from build123d import *

# Parameters (mm, degrees)
EXTRUDE_1_DEPTH     = 3
FILLET_1_R          = 1
EXTRUDE_2_DEPTH     = 12
EXTRUDE_2_TAPER     = 3
FILLET_3_R          = 3
FILLET_4_R          = 3
CUT_EXTRUDE_1_DEPTH = 2.54
SKETCH_5_W          = 0.63
SKETCH_5_H          = 0.63
EXTRUDE_3_DEPTH     = 2.54
CHAMFER_2_SIZE      = 0.2
CHAMFER_3_SIZE      = 0.2
CUT_EXTRUDE_2_DEPTH = 5.08
EXTRUDE_4_DEPTH     = 2.54
SKETCH_8_R          = 1.5
CUT_EXTRUDE_3_DEPTH = 0.1


with BuildPart() as part:
    # 草图1 → 凸台-拉伸1 (new body)
    with BuildSketch(Plane(origin=(0, 0, 0), x_dir=(1, 0, 0), z_dir=(0, 1, 0))):
        with BuildLine():
            ThreePointArc((11.109578501, 22.761132302), (9.268225449, 24.866230509), (6.58350481, 25.65))
            Line((6.58350481, 25.65), (-6.58350481, 25.65))
            ThreePointArc((-6.58350481, 25.65), (-9.268225449, 24.866230509), (-11.109578501, 22.761132302))
            Line((-11.109578501, 22.761132302), (-12.92017347, 18.860908481))
            ThreePointArc((-12.92017347, 18.860908481), (-13.440232827, 18.25183334), (-14.200505299, 18))
            ThreePointArc((-14.200505299, 18), (-16.897924527, 16.767729012), (-18, 14.014550498))
            Line((-18, 14.014550498), (-18, 13.985449502))
            Line((-18, 13.985449502), (-18, -13.985449502))
            Line((-18, -13.985449502), (-18, -14.014550498))
            ThreePointArc((-18, -14.014550498), (-16.897924527, -16.767729012), (-14.200505299, -18))
            ThreePointArc((-14.200505299, -18), (-13.440232827, -18.25183334), (-12.92017347, -18.860908481))
            Line((-12.92017347, -18.860908481), (-11.109578501, -22.761132302))
            ThreePointArc((-11.109578501, -22.761132302), (-9.268225449, -24.866230509), (-6.58350481, -25.65))
            Line((-6.58350481, -25.65), (6.58350481, -25.65))
            ThreePointArc((6.58350481, -25.65), (9.268225449, -24.866230509), (11.109578501, -22.761132302))
            Line((11.109578501, -22.761132302), (12.92017347, -18.860908481))
            ThreePointArc((12.92017347, -18.860908481), (13.440232827, -18.25183334), (14.200505299, -18))
            ThreePointArc((14.200505299, -18), (16.897924527, -16.767729012), (18, -14.014550498))
            Line((18, -14.014550498), (18, 14.014550498))
            ThreePointArc((18, 14.014550498), (16.897924527, 16.767729012), (14.200505299, 18))
            ThreePointArc((14.200505299, 18), (13.440232827, 18.25183334), (12.92017347, 18.860908481))
            Line((12.92017347, 18.860908481), (11.109578501, 22.761132302))
        make_face()
        with BuildLine():
            Line((6, -23.15), (-6, -23.15))
            ThreePointArc((-6, -23.15), (-7.5, -21.65), (-6, -20.15))
            Line((-6, -20.15), (6, -20.15))
            ThreePointArc((6, -20.15), (7.5, -21.65), (6, -23.15))
        make_face(mode=Mode.SUBTRACT)
        with BuildLine():
            ThreePointArc((-6, 20.15), (-7.5, 21.65), (-6, 23.15))
            Line((-6, 23.15), (6, 23.15))
            ThreePointArc((6, 23.15), (7.5, 21.65), (6, 20.15))
            Line((6, 20.15), (-6, 20.15))
        make_face(mode=Mode.SUBTRACT)
    extrude(amount=EXTRUDE_1_DEPTH)

    # 圆角1
    fillet_1_edges = [part.edges().sort_by_distance(p)[0] for p in [
        (-12.014875986, 3, 20.811020391),
        (-9.268225449, 3, 24.866230509),
        (0, 3, 25.65),
        (9.268225449, 3, 24.866230509),
        (12.014875986, 3, 20.811020391),
        (13.440232827, 3, 18.25183334),
        (16.897924527, 3, 16.767729012),
        (18, 3, 0),
        (16.897924527, 3, -16.767729012),
        (13.440232827, 3, -18.25183334),
        (12.014875986, 3, -20.811020391),
        (9.268225449, 3, -24.866230509),
        (0, 3, -25.65),
        (-9.268225449, 3, -24.866230509),
        (-12.014875986, 3, -20.811020391),
        (-13.440232827, 3, -18.25183334),
        (-16.897924527, 3, -16.767729012),
        (-18, 3, 0),
        (-16.897924527, 3, 16.767729012),
        (-13.440232827, 3, 18.25183334),
    ]]
    fillet(fillet_1_edges, radius=FILLET_1_R)

    # 草图2 → 凸台-拉伸2 (add)
    with BuildSketch(Plane(origin=(0, 3, 0), x_dir=(1, 0, 0), z_dir=(0, 1, 0))):
        with BuildLine():
            ThreePointArc((-14.15275961, 17.001140476), (-16.174133919, 16.077709334), (-17, 14.014550498))
            Line((-17, 14.014550498), (-17, -14.014550498))
            ThreePointArc((-17, -14.014550498), (-16.174133919, -16.077709334), (-14.15275961, -17.001140476))
            Line((-14.15275961, -17.001140476), (14.15275961, -17.001140476))
            ThreePointArc((14.15275961, -17.001140476), (16.174133919, -16.077709334), (17, -14.014550498))
            Line((17, -14.014550498), (17, 14.014550498))
            ThreePointArc((17, 14.014550498), (16.174133919, 16.077709334), (14.15275961, 17.001140476))
            Line((14.15275961, 17.001140476), (-14.15275961, 17.001140476))
        make_face()
    extrude(amount=EXTRUDE_2_DEPTH, taper=EXTRUDE_2_TAPER)

    # 圆角3
    # the kernel refuses this fillet: 3 mm, written as the material it takes off along each edge
    with BuildSketch(Plane(origin=(-21.254085444, 15, 16.372247124), x_dir=(0, 0, -1), z_dir=(1, 0, 0))) as fillet_3_piece_1:
        with BuildLine():
            CenterArc((FILLET_3_R * 0.948964566715, -FILLET_3_R), FILLET_3_R, 90, 87)
            Line((-FILLET_3_R * 0.0496649680397, -FILLET_3_R * 0.947664043757), (0, 0))
            Line((0, 0), (FILLET_3_R * 0.948964566715, 0))
        make_face()
    extrude(amount=42.508170888, mode=Mode.SUBTRACT)
    with BuildSketch(Plane(origin=(21.254085444, 15, -16.372247124), x_dir=(0, -0.9986295347545739, -0.05233595624294369), z_dir=(-1, 0, 0))) as fillet_3_piece_2:
        with BuildLine():
            CenterArc((FILLET_3_R * 0.948964566715, FILLET_3_R), FILLET_3_R, 183, 87)
            Line((-FILLET_3_R * 0.0496649680397, FILLET_3_R * 0.947664043757), (0, 0))
            Line((0, 0), (FILLET_3_R * 0.948964566715, 0))
        make_face()
    extrude(amount=42.508170888, mode=Mode.SUBTRACT)

    # 圆角4
    # the kernel refuses this fillet: 3 mm, written as the material it takes off along each edge
    with BuildSketch(Plane(origin=(-16.371106649, 15, -20.642587675), x_dir=(-0.052335956242944966, -0.9986295347545738, 0), z_dir=(0, 0, 1)), Plane(origin=(16.371106649, 15, 20.642587675), x_dir=(0.05233595624294368, -0.9986295347545738, 0), z_dir=(0, 0, -1))) as fillet_4_piece_1:
        with BuildLine():
            CenterArc((FILLET_4_R * 0.948964566715, FILLET_4_R), FILLET_4_R, 183, 87)
            Line((-FILLET_4_R * 0.0496649680397, FILLET_4_R * 0.947664043757), (0, 0))
            Line((0, 0), (FILLET_4_R * 0.948964566715, 0))
        make_face()
    extrude(amount=41.285175349, mode=Mode.SUBTRACT)

    # 草图4 → 切除-拉伸1 (cut)
    with BuildSketch(Plane(origin=(17.110228806, 0.896709095, 0), x_dir=(0, 0, -1), z_dir=(0.998629534754574, 0.05233595624294391, 0))):
        with BuildLine():
            Line((-5.1, 8.106177348), (5.1, 8.106177348))
            ThreePointArc((5.1, 8.106177348), (6.6, 6.606177348), (5.1, 5.106177348))
            Line((5.1, 5.106177348), (-5.1, 5.106177348))
            ThreePointArc((-5.1, 5.106177348), (-6.6, 6.606177348), (-5.1, 8.106177348))
        make_face()
    extrude(amount=-CUT_EXTRUDE_1_DEPTH, mode=Mode.SUBTRACT)

    # 草图5 → 凸台-拉伸3 (add)
    with BuildSketch(Plane(origin=(14.573709787, 0.763775766, 0), x_dir=(0, 0, -1), z_dir=(0.998629534754574, 0.05233595624294393, 0))):
        with Locations((-1.27, 6.606177348)):
            Rectangle(SKETCH_5_W, SKETCH_5_H)
        with Locations((-3.81, 6.606177348)):
            Rectangle(SKETCH_5_W, SKETCH_5_H)
        with Locations((1.27, 6.606177348)):
            Rectangle(SKETCH_5_W, SKETCH_5_H)
        with Locations((3.81, 6.606177348)):
            Rectangle(SKETCH_5_W, SKETCH_5_H)
    extrude(amount=EXTRUDE_3_DEPTH)

    # 倒角2
    chamfer_2_edges = [part.edges().sort_by_distance(p)[0] for p in [
        (16.780974023, 7.179264603, 3.81),
        (16.764488197, 7.493832906, 4.125),
        (16.748002371, 7.80840121, 3.81),
        (16.764488197, 7.493832906, 3.495),
    ]]
    chamfer(chamfer_2_edges, length=CHAMFER_2_SIZE)

    # 倒角3
    chamfer_3_edges = [part.edges().sort_by_distance(p)[0] for p in [
        (16.764488197, 7.493832906, 1.585),
        (16.748002371, 7.80840121, 1.27),
        (16.764488197, 7.493832906, 0.955),
        (16.780974023, 7.179264603, 1.27),
        (16.764488197, 7.493832906, -0.955),
        (16.748002371, 7.80840121, -1.27),
        (16.764488197, 7.493832906, -1.585),
        (16.780974023, 7.179264603, -1.27),
        (16.764488197, 7.493832906, -3.495),
        (16.748002371, 7.80840121, -3.81),
        (16.764488197, 7.493832906, -4.125),
        (16.780974023, 7.179264603, -3.81),
    ]]
    chamfer(chamfer_3_edges, length=CHAMFER_3_SIZE)

    # 草图6 → 切除-拉伸2 (cut)
    with BuildSketch(Plane(origin=(-17.110228806, 0.896709095, 0), x_dir=(0, 0, 1), z_dir=(-0.998629534754574, 0.05233595624294391, -1.6069369669372317e-15))):
        with BuildLine():
            Line((-2.9, 7.606177348), (2.9, 7.606177348))
            ThreePointArc((2.9, 7.606177348), (4.15, 6.356177348), (2.9, 5.106177348))
            Line((2.9, 5.106177348), (-2.9, 5.106177348))
            ThreePointArc((-2.9, 5.106177348), (-4.15, 6.356177348), (-2.9, 7.606177348))
        make_face()
    extrude(amount=-CUT_EXTRUDE_2_DEPTH, mode=Mode.SUBTRACT)

    # 草图7 → 凸台-拉伸4 (add)
    with BuildSketch(Plane(origin=(-12.037190769, 0.630842437, 0), x_dir=(0, 0, 1), z_dir=(-0.998629534754574, 0.05233595624294393, -1.6069369669372323e-15))):
        with BuildLine():
            Line((-2.5, 6.431177348), (2.5, 6.431177348))
            ThreePointArc((2.5, 6.431177348), (2.575, 6.356177348), (2.5, 6.281177348))
            Line((2.5, 6.281177348), (-2.5, 6.281177348))
            ThreePointArc((-2.5, 6.281177348), (-2.575, 6.356177348), (-2.5, 6.431177348))
        make_face()
    extrude(amount=EXTRUDE_4_DEPTH)

    # 草图8 → 切除-拉伸3 (cut)
    with BuildSketch(Plane.XZ):
        with Locations(Location((14.01, 14.014550498, 0), (0, 0, 270))):
            Circle(SKETCH_8_R)
        with Locations(Location((-14.01, -14.014550498, 0), (0, 0, 270))):
            Circle(SKETCH_8_R)
    extrude(amount=-CUT_EXTRUDE_3_DEPTH, mode=Mode.SUBTRACT)


solid = part.part
Check sheet for the modelled part. Datum: model origin and axes. Units: mm. A direction names the side the tool comes from. Coordinates: 2 decimals unless noted, no trailing zeros. Answer in a Markdown table with one row per item.
1. Material ranges on line 1 along Y through (x, z) = (0.5, -15.5); line 2 along X through (y, z) = (8, 3); line 3 along X through (y, z) = (6, -11.5), recorded low to high. Write a range as [from, to].
Check values:
| item | result |
|---|---|
| line 1 | y = [0, 14.26] |
| line 2 | x = [-11.65, 14.19] |
| line 3 | x = [-16.84, 16.84] |
2. Sectioned sample at A-A, the plane x = -4.5. Give the number of separate pieces and of enclosed holes in the cut face, then the cut area to 3 significant figures.
Check values:
| item | result |
|---|---|
| separate pieces | 3 |
| enclosed holes | 0 |
| area | 533 mm2 |
3. Go/stop test with flat-tipped pins: pin 1 (8 mm diameter, centred on y = 9, z = -6.5, fed in from -X); pin 2 (0.6 mm diameter, centred on x = 15.5, y = 7.5, fed in from -Z); pin 3 (3 mm diameter, centred on x = 6.5, y = 6, fed in from +Z). Record where each tip stops, or that it passes through.
Check values:
| item | result |
|---|---|
| pin 1 | stops at x = -16.9 |
| pin 2 | stops at z = -16.5 |
| pin 3 | stops at z = 16.92 |
4. Release check for a two-part mould opening along Z. For faces 1 (the face through (9.302, 0.986, -24.845)), 2 (the face through (-12.03, 0.99, 20.78)), 3 (the face through (0, 1, 20.15)) record: released by +Z, released by -Z, zero draft, split by the parting line, or undercut.
Check values:
| item | result |
|---|---|
| face 1 | released by -Z |
| face 2 | released by +Z |
| face 3 | undercut |
5. Access from +Z, -Z, +X, -X, +Y, -Y to the whole of each face (thin tool, end or side, straight path). Record for faces 4 (the face through (-12.95, 7.12, -0.04)), 5 (the face through (0, 1, 23.15)), 6 (the face through (-0.2, 3, 19.9)).
Check values:
| item | result |
|---|---|
| face 4 | none |
| face 5 | +Y, -Y |
| face 6 | +Z, +X, -X, +Y |
